Build history of the part. All positions in model axes, mm. Face numbers are marked on the shaded views. Round coordinates to 2 decimals unless told otherwise and drop trailing zeros. Write each loop counter-clockwise with the first axis right and the second up, starting at its lowest first coordinate (ties: lowest second). Pieces come first, ordered by that corner, then holes. Notation, with made-up numbers: (53.5, 58.25) - (69.5, 58.25) arc R28 ccw to (69.5, 86.25) - close; hole circle Ø3 at (73.25, 47.25). An arc over 180 degrees is marked (long way). One line per question, with ' | ' between items.
from build123d import *

# Parameters (mm, degrees)
SKETCH2_W   = 1.982852704
SKETCH2_H   = 4.045354148
SKETCH2_W_2 = 0.933543265
SKETCH2_H_2 = 4.667716324
SKETCH2_W_3 = 1.011338537


with BuildPart() as part:
    # Sketch1 → Revolve1 (revolve)
    with BuildSketch(Plane.XY, mode=Mode.PRIVATE) as revolve1_sk:
        with BuildLine():
            Line((-10.091533181, 57.356979405), (-10.091533181, 45))
            Line((-10.091533181, 45), (10.091533181, 45))
            Line((10.091533181, 45), (10.091533181, 57.356979405))
            ThreePointArc((10.091533181, 57.356979405), (0, 67.448512586), (-10.091533181, 57.356979405))
        make_face()
    revolve(revolve1_sk.sketch.rotate(Axis((-52.285660481, 0, 0), (1, 0, 0)), 90), axis=Axis((-52.285660481, 0, 0), (1, 0, 0)))

    # Sketch2 → Cut-Revolve1 (revolve, cut)
    with BuildSketch(Plane.XY, mode=Mode.PRIVATE) as cut_revolve1_sk:
        with Locations((0, 68.723356154)):
            Rectangle(SKETCH2_W, SKETCH2_H)
        with Locations((2.937234888, 68.723356154)):
            Rectangle(SKETCH2_W_2, SKETCH2_H_2)
        with Locations((-3.286386879, 68.723356154)):
            Rectangle(SKETCH2_W_3, SKETCH2_H_2)
    revolve(cut_revolve1_sk.sketch.rotate(Axis((38.367575356, 0, 0), (1, 0, 0)), 90), axis=Axis((38.367575356, 0, 0), (1, 0, 0)), mode=Mode.SUBTRACT)


solid = part.part
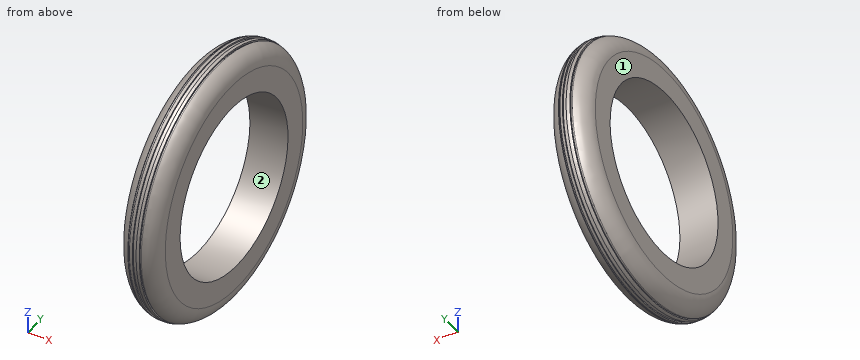
Q1. Drop flat-ended pins along their axis: pin 1 (6 mm diameter, centred on x = -1.5, z = -31, fed in from -Y); pin 2 (5 mm diameter, centred on x = 1, z = 48, fed in from -Y); pin 3 (12 mm diameter, centred on x = 0.5, y = 31.5, fed in from -Z). Give the stop position or say it passes through.
Found:
pin 1: y = -61.29 | pin 2: y = -49.72 | pin 3: z = -62.38
Q2. Saw through at C-C, the plane x = 7. List the corners of the cut face in (y, z), then the cut area to 3 significant figures.
Found:
outline: circle Ø129.25 at (0, 0); hole circle Ø90 at (0, 0) | area: 6,760 mm^2
Q3. Drill centre lines: L1, parallel to Y at x = 0, z = 0; L2, parallel to Z at x = 8.75, y = 21; L3, parallel to Z at x = 0, y = -7. Where is each one in solid material? Low to high. Write a range as from..to.
Found:
L1: -66.7..-45, 45..66.7 | L2: -58.74..-39.8, 39.8..58.74 | L3: -66.33..-44.45, 44.45..66.33
Q4. Pull direction Z, two halves, no side cores. Call the marked faces 1 and 2: +Z half, -Z half, draft (parallel to the pull), parting line (faces both ways), or undercut.
Found:
face 1: draft | face 2: undercut
